```python
from build123d import *

# Parameters (mm, degrees)
CUT_EXTRUDE2_DEPTH = 120


with BuildPart() as part:
    # Sketch1 → Revolve1 (revolve)
    with BuildSketch(Plane(origin=(0, 0, 0), x_dir=(1, 0, 0), z_dir=(0, 1, 0)), mode=Mode.PRIVATE) as revolve1_sk:
        Polygon((-87.474048443, 20), (52.595155709, 20), (52.595155709, 30), (-39.474048443, 30), (-39.474048443, 40), (0.525951557, 40), (0.525951557, 52.948096886), (40.525951557, 52.948096886), (40.525951557, 62.948096886), (72.525951557, 62.948096886), (72.525951557, 78.546712803), (32.525951557, 78.546712803), (32.525951557, 60), (-7.474048443, 60), (-7.474048443, 50), (-47.474048443, 50), (-47.474048443, 40), (-87.474048443, 40), align=None)
    revolve(revolve1_sk.sketch.rotate(Axis((-87.474048443, 0, 0), (1, 0, 0)), 180), axis=Axis((-87.474048443, 0, 0), (1, 0, 0)))

    # Sketch2 → Cut-Extrude2 (cut)
    with BuildSketch(Plane.ZY.offset(87.474048443)):
        Polygon((-3.470245106, -25.786795459), (-3.470245106, -19.696634202), (6.863316134, -18.785496843), (6.863316134, -25.786795459), align=None)
    extrude(amount=-CUT_EXTRUDE2_DEPTH, mode=Mode.SUBTRACT)


solid = part.part
```
Can you work these out from the model? Positions are in its coordinate system, mm. A direction names the side the tool comes from. Give positions to 0.01 mm unless a question says otherwise; leave off trailing zeros. Write each loop counter-clockwise with the first axis right and the second up, starting at its lowest first coordinate (ties: lowest second). Pieces come first, ordered by that corner, then holes. Notation, with made-up numbers: (-2, 52.25) -> (28, 52.25) arc R30 ccw to (28, 85.25) -> close; hole circle Ø9 at (75, 31). An arc over 180 degrees is marked (long way). Write item = value, one per line.
(1) Suppose I cut it at D-D on y = 66. Write out the boundary of the cut face in (x, z).
Worked out:
outline = (32.53, -42.59) -> (72.53, -42.59) -> (72.53, 42.59) -> (32.53, 42.59) -> close
(2) Suppose I cut it at B-B on x = -69.5. Write out the boundary of the cut face in (y, z), then the cut area to 3 significant figures.
Worked out:
outline = circle Ø80 at (0, 0); hole (-25.79, -3.47) -> (-19.7, -3.47) arc R20 ccw (long way) to (-18.79, 6.86) -> (-25.79, 6.86) -> close
area = 3,710 mm^2
(3) Suppose I cut it at A-A on x = -22. Write out the boundary of the cut face in (y, z), then the cut area to 3 significant figures.
Worked out:
outline = circle Ø100 at (0, 0); circle Ø60 at (0, 0); hole circle Ø80 at (0, 0); hole (-25.79, -3.47) -> (-19.7, -3.47) arc R20 ccw (long way) to (-18.79, 6.86) -> (-25.79, 6.86) -> close
area = 4,340 mm^2
(4) For faces 4 (the face through (-28, -22, 6.863)), 5 (the face through (72.526, -24, 59)), 6 (the face through (40.526, -52, 14)), which set-ups out of +Z, -Z, +X, -X, +Y, -Y let a thin tool reach every point of the face, with its end or its side?
Worked out:
face_4 = -X
face_5 = +Z, -Z, +X, +Y, -Y
face_6 = +X
(5) I'm going to push flat-ended pins straight in: P1, Ø8.5, axis at x = -44, z = 2.5, coming from the +Y side; P2, Ø8, axis at x = 24.5, y = 32.5, coming from the +Z side; P3, Ø6, axis at x = -61, z = 29, coming from the +Y side; P4, Ø24, axis at y = 0, z = 0, coming from the -X side. Where does each tip first touch, or does it pass through?
Worked out:
P1 = 50
P2 = 52.8
P3 = 30.4
P4 = through
(6) Suppose I cut it at C-C on z = 47.5. Write out the boundary of the cut face in (x, y).
Worked out:
outline = (-47.47, -15.61) -> (-7.47, -15.61) -> (-7.47, -36.66) -> (32.53, -36.66) -> (32.53, -62.56) -> (72.53, -62.56) -> (72.53, -41.31) -> (40.53, -41.31) -> (40.53, -23.39) -> (0.53, -23.39) -> (0.53, 23.39) -> (40.53, 23.39) -> (40.53, 41.31) -> (72.53, 41.31) -> (72.53, 62.56) -> (32.53, 62.56) -> (32.53, 36.66) -> (-7.47, 36.66) -> (-7.47, 15.61) -> (-47.47, 15.61) -> close
(7) I need wall thicknesses on probe 1 along Y at (x, z) = (-14, 0); probe 2 along Y at (x, z) = (62, 0); probe 3 along Z at (x, y) = (-21.5, 1). Which ranges of each line are inside material? Lowest first, please. Write a range as from..to.
Worked out:
probe_1 = -50..-40, -30..-25.79, 20..30, 40..50
probe_2 = -78.55..-62.95, 62.95..78.55
probe_3 = -49.99..-39.99, -29.98..-19.97, 19.97..29.98, 39.99..49.99
(8) Thinking about a two-plate mould opening in Y: for faces 1 (the face through (-7.474, -45, -23)), 2 (the face through (-16.459, 19.524, -4.336)), 3 (the face through (-67.75, -1.76, -39.96)), which applies, released by +Y, released by -Y, zero draft, split by the parting line, or undercut?
Worked out:
face_1 = zero draft
face_2 = undercut
face_3 = split by the parting line
